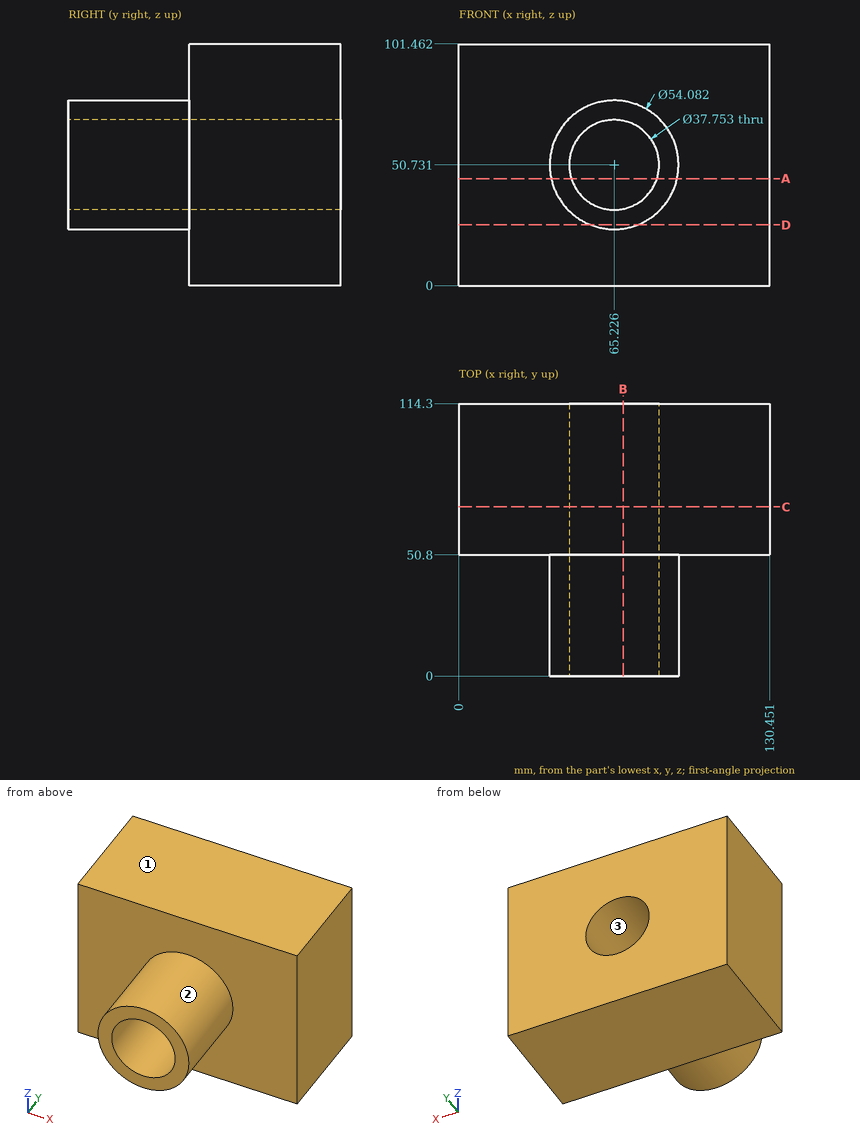
Geometry check sheet. Reference: drawing and pictorial views, mm from the part's lowest x, y, z. Coordinates: 2 decimals unless noted, no trailing zeros. Order: outer loops, then holes, each group sorted by start corner. A loop starts at its lowest first (then second) coordinate and runs counter-clockwise, first axis right, second up. Notation, with made-up numbers: (37, -10.5) - (44, -10.5) arc R10 cw to (44, 1.5) - close; hole circle Ø8 at (29, 68.5). An arc over 180 degrees is marked (long way). One line per item, written item: value.
(1) Thickness scan on probe 1 along Y at (x, z) = (35, 77.5); probe 2 along Z at (x, y) = (81, 84) (1 decimal); probe 3 along X at (y, z) = (79.5, 55). Record the ranges inside material, lowest first. Write a range as from..to.
Data:
probe 1: y = 50.8..114.3
probe 2: z = 0..40.4, 61.1..101.5
probe 3: x = 0..46.84, 83.61..130.45
(2) Sectioned sample at A-A (z = 45). Enter the section's corners in (x, y), and give its area (3 significant figures).
Data:
outline: (0, 50.8) - (38.8, 50.8) - (38.8, 0) - (47.24, 0) - (47.24, 114.3) - (0, 114.3) - close; (83.21, 0) - (91.65, 0) - (91.65, 50.8) - (130.45, 50.8) - (130.45, 114.3) - (83.21, 114.3) - close
area: 6,860 mm^2
(3) Sectioned sample at D-D (z = 25.5). Enter the section's corners in (x, y), and give its area (3 significant figures).
Data:
outline: (0, 50.8) - (55.5, 50.8) - (55.5, 0) - (74.95, 0) - (74.95, 50.8) - (130.45, 50.8) - (130.45, 114.3) - (0, 114.3) - close
area: 9,270 mm^2
(4) Sectioned sample at C-C (y = 71). Enter the section's corners in (x, z) (1 decimal).
Data:
outline: (0, 0) - (130.5, 0) - (130.5, 101.5) - (0, 101.5) - close; hole circle Ø37.8 at (65.2, 50.7)
(5) Sectioned sample at B-B (x = 69). Enter the section's corners in (y, z) (1 decimal).
Data:
outline: (0, 24) - (50.8, 24) - (50.8, 0) - (114.3, 0) - (114.3, 32.2) - (0, 32.2) - close; (0, 69.2) - (114.3, 69.2) - (114.3, 101.5) - (50.8, 101.5) - (50.8, 77.5) - (0, 77.5) - close
(6) Release check for a two-part mould opening along X. For the marked faces 1, 2 and 3 record: +X half, -X half, draft (parallel to the pull), parting line (faces both ways), or undercut.
Data:
face 1: draft
face 2: parting line
face 3: undercut
(7) Depth check by flat-ended pin: pin 1 Ø3 at (x, y) = (65, 34.5) entering from -Z; pin 2 Ø10 at (y, z) = (53.5, 46.5) entering from -X; pin 3 Ø1.5 at (x, z) = (109.5, 16.5) entering from -Y. Enter the tip coordinate at first touch or a pass-through.
Data:
pin 1: stops at z = 23.69
pin 2: stops at x = 0
pin 3: stops at y = 50.8
